Work out the finished part from the listing and answer in its coordinate system (mm). Give positions to 0.01 mm unless a question says otherwise; leave off trailing zeros. Write each loop counter-clockwise with the first axis right and the second up, starting at its lowest first coordinate (ties: lowest second). Pieces come first, ordered by that corner, then holes.
1) Find section B-B (x = 54). Determine the outline of the cut face in (y, z) (3 decimals), plus the area to 3 significant figures.
2) Straight lines are drawn through the part: probe 1 along X at (y, z) = (2.15, -560) (3 decimals); probe 2 along Z at (x, y) = (73.5, 1.95) (3 decimals). For each, find the intervals that lie inside material, in ascending order.
3) Given pin 1 Ø0.8 at (y, z) = (1, -23.5) entering from +X; pin 2 Ø0.8 at (x, y) = (61, 1) entering from -Z (3 decimals); pin 3 Ø1.5 at (x, y) = (55.5, 0.5) entering from +Z (3 decimals), each flat-ended and moving along its own axis, determine where each tip first touches the part or whether it passes through.
```python
from build123d import *

# Parameters (mm, degrees)
SKETCH1_W           = 190.5
SKETCH1_H           = 609.6
BOSS_EXTRUDE1_DEPTH = 2.778125
SKETCH2_W           = 190.5
SKETCH2_H           = 17.78
CUT_EXTRUDE1_DEPTH  = 3.778125
SKETCH3_W           = 17.78
SKETCH3_H           = 574.04
CUT_EXTRUDE2_DEPTH  = 3.778125
SKETCH4_W           = 10.16
SKETCH4_H           = 10.16
CUT_EXTRUDE3_DEPTH  = 3.778125
FILLET1_R           = 2.54


with BuildPart() as part:
    # Sketch1 → Boss-Extrude1 (new body)
    with BuildSketch(Plane(origin=(0, 0, 0), x_dir=(1, 0, 0), z_dir=(0, 1, 0))):
        with Locations((95.25, 304.8)):
            Rectangle(SKETCH1_W, SKETCH1_H)
    extrude(amount=BOSS_EXTRUDE1_DEPTH)

    # Sketch2 → Cut-Extrude1 (cut, through all)
    with BuildSketch(Plane(origin=(0, 2.778125, 0), x_dir=(1, 0, 0), z_dir=(0, 1, 0))):
        with Locations((95.25, 8.89)):
            Rectangle(SKETCH2_W, SKETCH2_H)
        with Locations((95.25, 600.71)):
            Rectangle(SKETCH2_W, SKETCH2_H)
    extrude(amount=-CUT_EXTRUDE1_DEPTH, mode=Mode.SUBTRACT)

    # Sketch3 → Cut-Extrude2 (cut, through all)
    with BuildSketch(Plane(origin=(0, 2.778125, 0), x_dir=(1, 0, 0), z_dir=(0, 1, 0))):
        with Locations((8.89, 304.8)):
            Rectangle(SKETCH3_W, SKETCH3_H)
    extrude(amount=-CUT_EXTRUDE2_DEPTH, mode=Mode.SUBTRACT)

    # Sketch4 → Cut-Extrude3 (cut, through all)
    with BuildSketch(Plane(origin=(0, 2.778125, 0), x_dir=(1, 0, 0), z_dir=(0, 1, 0))):
        Polygon((17.78, 591.82), (76.454, 591.82), (76.454, 574.675), (27.305, 574.675), (27.305, 533.146), (17.78, 533.146), align=None)
        Polygon((17.78, 17.78), (76.454, 17.78), (76.454, 34.925), (27.305, 34.925), (27.305, 76.454), (17.78, 76.454), align=None)
        with Locations((185.42, 586.74)):
            Rectangle(SKETCH4_W, SKETCH4_H)
        with Locations((185.42, 22.86)):
            Rectangle(SKETCH4_W, SKETCH4_H)
    extrude(amount=-CUT_EXTRUDE3_DEPTH, mode=Mode.SUBTRACT)

    # Fillet1
    fillet1_edges = [part.edges().sort_by_distance(p)[0] for p in [
        (17.78, 1.3890625, -76.454),
        (27.305, 1.3890625, -76.454),
        (27.305, 1.3890625, -34.925),
        (76.454, 1.3890625, -34.925),
        (76.454, 1.3890625, -17.78),
        (190.5, 1.3890625, -581.66),
        (180.34, 1.3890625, -591.82),
        (190.5, 1.3890625, -27.94),
        (180.34, 1.3890625, -17.78),
        (17.78, 1.3890625, -533.146),
        (76.454, 1.3890625, -591.82),
        (76.454, 1.3890625, -574.675),
        (27.305, 1.3890625, -574.675),
        (27.305, 1.3890625, -533.146),
    ]]
    fillet(fillet1_edges, radius=FILLET1_R)


solid = part.part
```
Results:
1. outline: (0, -574.675) - (2.778, -574.675) - (2.778, -34.925) - (0, -34.925) - close
1. area: 1,500 mm2
2. probe 1: x = 27.305 to 190.5
2. probe 2: z = -574.675 to -34.925
3. pin 1: stops at x = 180.34
3. pin 2: stops at z = -574.675
3. pin 3: stops at z = -34.925
